Autodesk Inventor part; units mm, degrees
ref_plane "YZ Plane" through (0, 0, 0) normal (1, 0, 0) x (0, 1, 0)
ref_plane "XZ Plane" through (0, 0, 0) normal (0, 1, 0) x (-1, 0, 0)
ref_plane "XY Plane" through (0, 0, 0) normal (0, 0, 1) x (1, 0, 0)
sketch "Sketch3" plane through (0, 0, 0) normal (0, 1, 0) x (-1, 0, 0)
  line L0 (0, 0) -> (11, 0)
  line L1 (11, 0) -> (11, -56)
  line L2 (11, -56) -> (0, -56)
  line L3 (0, -56) -> (0, 0)
  line L4 (12, 1) -> (-1, 1)
  line L5 (-1, 1) -> (-1, -57)
  line L6 (-1, -57) -> (12, -57)
  line L7 (12, -57) -> (12, 1)
  line L8 (7.5, -6.2) -> (3.5, -6.2)
  line L9 (1.5, -8.2) -> (1.5, -12)
  line L10 (3.5, -14) -> (7.5, -14)
  line L11 (9.5, -12) -> (9.5, -8.2)
  arc A0 (9.5, -8.2) -> (7.5, -6.2) centre (7.5, -8.2) ccw
  arc A1 (7.5, -14) -> (9.5, -12) centre (7.5, -12) ccw
  arc A2 (1.5, -12) -> (3.5, -14) centre (3.5, -12) ccw
  arc A3 (3.5, -6.2) -> (1.5, -8.2) centre (3.5, -8.2) ccw
  circle A4 centre (5.5, -51) radius 1
  point P0 (1.5, -14)
  point P1 (1.5, -6.2)
  point P2 (9.5, -14)
  dimension "d2" = 11
  dimension "d3" = 56
  dimension "d4" = 1
  dimension "d5" = 1
  dimension "d6" = 1
  dimension "d7" = 1
  dimension "d8" = 8
  dimension "d9" = 7.8
  dimension "d10" = 14
  dimension "d11" = 9.5
  dimension "d12" = 2
  dimension "d30" = 2
  dimension "d31" = 5
  dimension "d32" = 5.5
extrude "Extrusion1" add sketch "Sketch3" along normal blind 1.4 contours L0 L1 L2 L3
extrude "Extrusion3" add sketch "Sketch3" along normal blind 8.6 contours L7 L6 L5 L4
sketch "Sketch4" plane through (-12, 0, 1) normal (0, 0, 1) x (1, 0, 0)
  circle A0 centre (6.5, 5.4) radius 2.65
  line L0 (0, 0) -> (0, 8.6)
  line L1 (0, 0) -> (13, 0)
  point P0 (12, 0)
  dimension "d19" = 6.5
  dimension "d20" = 5.3
  dimension "d21" = 5.4
extrude "Extrusion4" cut sketch "Sketch4" against normal blind 8.6
sketch "Sketch5" plane through (1, 0, -57) normal (0, 0, -1) x (-1, 0, 0)
  line L0 (2.675, 6.25) -> (10.325, 6.25)
  line L1 (10.325, 6.25) -> (10.325, 3.55)
  line L2 (10.325, 3.55) -> (2.675, 3.55)
  line L3 (2.675, 3.55) -> (2.675, 6.25)
  line L4 (0, 0) -> (13, 0)
  line L5 (13, 0) -> (13, 8.6)
  point P0 (1, 0)
  dimension "d24" = 7.65
  dimension "d25" = 2.7
  dimension "d26" = 3.55
  dimension "d27" = 2.675
extrude "Extrusion5" cut sketch "Sketch5" against normal blind 8.6
equation "\"d11\" = 0.5 * d2 + 0.5 * d8"
equation "\"d32\" = 0.5 * d2"
equation "\"d19\" = 0.5 * d2 + d4"
properties part number "QC25BTFication_1"
Geometry: final body of the model. Coordinates: model frame, mm. A direction names the side the tool comes from. Give positions to 0.01 mm unless a question says otherwise; leave off trailing zeros. Loops run counter-clockwise (first coordinate to the right, second up) from the corner with the lowest first, then second, coordinate; pieces in that order, holes last. Notation, with made-up numbers: (44, 81.5) - (74, 81.5) arc R30 cw to (74, 117.5) - close; hole circle Ø9 at (45, 30.25). An arc over 180 degrees is marked (long way). Answer as CSV lines item,"result". Start each with the question number.
1. Section A-A, the plane x = -5.5. Return loops of the section in (y, z).
2. Ray query, L1, parallel to X at y = 7.5, z = -33; L2, parallel to Y at x = -5.5, z = 0.4; L3, parallel to Z at x = -5.25, y = 1. Return the intervals inside material, ascending.
3. Draft query along X for faces 1 (the face through (-8.93, 0.69, -13.4)), 2 (the face through (-2.07, 0.69, -6.8)), 3 (the face through (-12, 4, -28)), 4 (the face through (-5, 3, -57)). Return one class per face: released by +X, released by -X, zero draft, split by the parting line, or undercut.
4. Section B-B, the plane z = -10. Return loops of the section in (x, y), plus the area to 3 significant figures.
5. Pin query (flat end, axial travel): P1, Ø1.1, axis at x = -7, z = -56.5, coming from the -Y side; P2, Ø5.5, axis at x = -3, z = -21.5, coming from the +Y side. Return the tip coordinate at first contact, or that it passes through.
6. Reachability of faces 5 (the face through (-1.675, 4.9, -56.5)), 6 (the face through (-5.84, 8.03, 0.51)), 7 (the face through (-1.5, 1, -10)), 8 (the face through (-5.4, 2.5, 0)) from +Z, -Z, +X, -X, +Y, -Y: full face, straight path, thin tool, end or side. Return the list, or none.
7. Section D-D, the plane y = 2. Return loops of the section in (x, z), plus the area to 3 significant figures.
8. Section C-C, the plane y = 5.4. Return loops of the section in (x, z) (3 decimals).
Answers:
1,outline,"(0, -57) - (3.55, -57) - (3.55, -56) - (1.4, -56) - (1.4, -52) - (0, -52) - close; (0, -50) - (1.4, -50) - (1.4, -14) - (0, -14) - close; (0, -6.2) - (1.4, -6.2) - (1.4, 0) - (2.75, 0) - (2.75, 1) - (0, 1) - close; (6.25, -57) - (8.6, -57) - (8.6, -56) - (6.25, -56) - close; (8.05, 0) - (8.6, 0) - (8.6, 1) - (8.05, 1) - close"
2,L1,"x = -12 to -11, 0 to 1"
2,L2,"y = 0 to 2.75, 8.05 to 8.6"
2,L3,"z = -57 to -51.97, -50.03 to -14, -6.2 to 1"
3,face 1,"undercut"
3,face 2,"undercut"
3,face 3,"released by -X"
3,face 4,"zero draft"
4,outline,"(-12, 0) - (-9.5, 0) - (-9.5, 1.4) - (-11, 1.4) - (-11, 8.6) - (-12, 8.6) - close; (-1.5, 0) - (1, 0) - (1, 8.6) - (0, 8.6) - (0, 1.4) - (-1.5, 1.4) - close"
4,area,"21.4 mm2"
5,P1,"stops at y = 0"
5,P2,"stops at y = 1.4"
6,face 5,"-Z"
6,face 6,"+Z"
6,face 7,"+Y, -Y"
6,face 8,"+Y"
7,outline,"(-12, -57) - (1, -57) - (1, 1) - (-12, 1) - close; hole (-11, -56) - (0, -56) - (0, 0) - (-11, 0) - close"
7,area,"138 mm2"
8,outline,"(-12, -57) - (-9.325, -57) - (-9.325, -56) - (-11, -56) - (-11, 0) - (-8.15, 0) - (-8.15, 1) - (-12, 1) - close; (-2.85, 0) - (0, 0) - (0, -56) - (-1.675, -56) - (-1.675, -57) - (1, -57) - (1, 1) - (-2.85, 1) - close"
